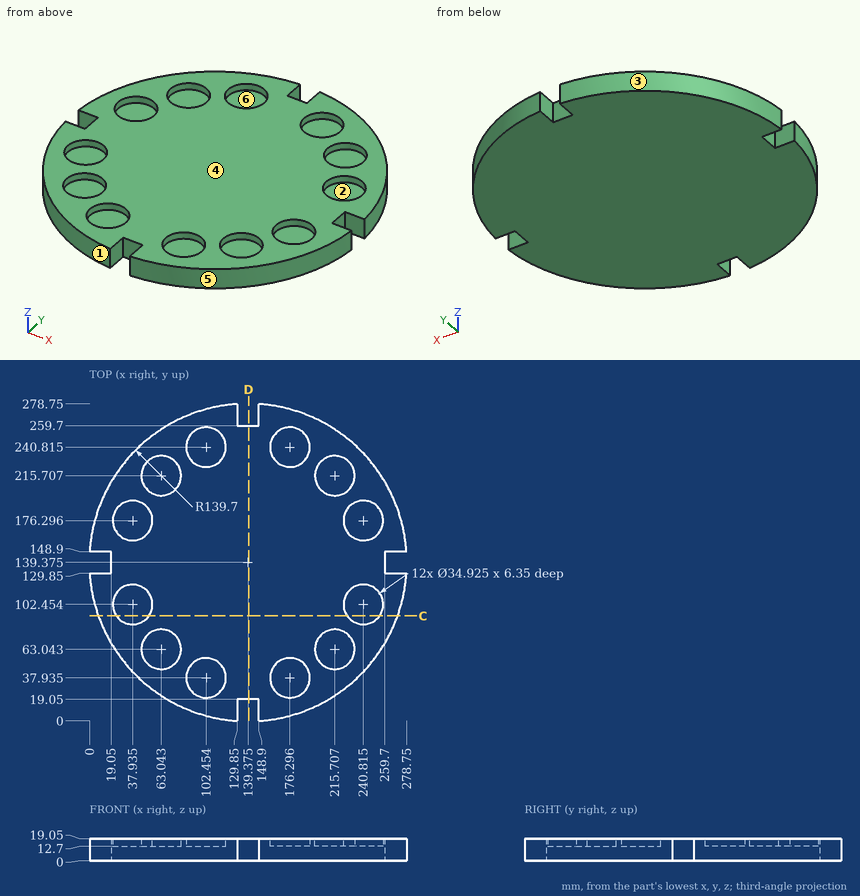
The figure shows three views and two pictorial views of one solid part (mm, origin at its lowest corner). Answer the questions. A direction names the side the tool comes from. Coordinates: 2 decimals unless noted, no trailing zeros. Loops run counter-clockwise (first coordinate to the right, second up) from the corner with the lowest first, then second, coordinate; pieces in that order, holes last. Notation, with made-up numbers: M -5,19 L 30,19 A20 ccw 30,41 Z; hole C 51.5,40 d4. An arc over 180 degrees is marked long. Answer as CSV lines item,"result". Start each with the question number.
(1) The mould has two halves that part along Y. Classify the marked faces 3, 4, 5 and 6: pulls with the +Y half, pulls with the -Y half, needs draft (parallel to the pull), parting line crosses it, or undercut.
(2) Find the intervals of material crossed by L1, parallel to Y at x = 109.5, z = 17; L2, parallel to Y at x = 216.5, z = 18.25 (1 decimal); L3, parallel to X at y = 174, z = 17 (1 decimal), in increasing order. Write a range as [from, to].
(3) The part is cut by section C-C (y = 92.5). Give the vertices of the cut face in (x, z).
(4) The part is cut by section D-D (x = 140). Give the vertices of the cut face in (y, z).
(5) For the marked faces 1 and 2, determine the directions among +Z, -Z, +X, -X, +Y, -Y from which every point of the face is accessible in a straight line to the end or side of a thin tool.
(6) Given pin 1 (5 mm diameter, centred on x = 197.5, z = 16, fed in from +Y); pin 2 (2 mm diameter, centred on x = 82, z = 6.5, fed in from +Y) (1 decimal); pin 3 (8 mm diameter, centred on x = 43, z = 7, fed in from -Y) (1 decimal), each flat-ended and moving along its own axis, determine where each tip first touches the part or whether it passes through.
Determined:
1,face 3,"pulls with the +Y half"
1,face 4,"needs draft"
1,face 5,"pulls with the -Y half"
1,face 6,"undercut"
2,L1,"[2.91, 21.96], [53.91, 224.84], [256.79, 275.84]"
2,L2,"[22.9, 45.6], [80.5, 198.3], [233.2, 255.9]"
2,L3,"[4, 20.6], [55.2, 223.5], [258.1, 274.7]"
3,outline,"M 7.77,0 L 270.98,0 L 270.98,19.05 L 255.16,19.05 L 255.16,12.7 L 226.47,12.7 L 226.47,19.05 L 52.28,19.05 L 52.28,12.7 L 23.59,12.7 L 23.59,19.05 L 7.77,19.05 Z"
4,outline,"M 19.05,0 L 259.7,0 L 259.7,19.05 L 19.05,19.05 Z"
5,face 1,"+Z, -Z, -X, -Y"
5,face 2,"+Z"
6,pin 1,"y = 267.52"
6,pin 2,"y = 267.2"
6,pin 3,"y = 34.6"
